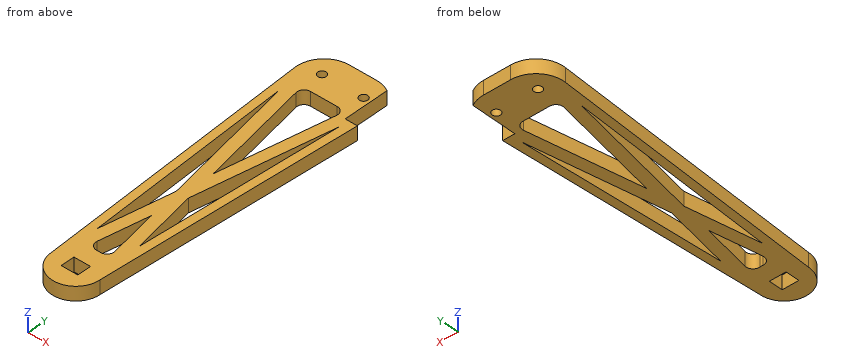
```python
from build123d import *

# Parameters (mm, degrees)
SKETCH1_R           = 3
BOSS_EXTRUDE2_DEPTH = 10
FILLET1_R           = 20
FILLET2_R           = 20
CUT_EXTRUDE1_START  = -10
CUT_EXTRUDE1_DEPTH  = 10
FILLET3_R           = 5
CUT_EXTRUDE6_DEPTH  = 10


with BuildPart() as part:
    # Sketch1 → Boss-Extrude2 (new body)
    with BuildSketch(Plane.XY):
        with BuildLine():
            Line((-30, 15.770412854), (-30, 0))
            Line((-30, 0), (-17.5, -210))
            ThreePointArc((-17.5, -210), (0, -227.5), (17.5, -210))
            Line((17.5, -210), (30, 0))
            Line((30, 0), (30, 15.770412854))
            Line((30, 15.770412854), (-30, 15.770412854))
        make_face()
        with Locations((-15, 0)):
            Circle(SKETCH1_R, mode=Mode.SUBTRACT)
        with Locations((15, 0)):
            Circle(SKETCH1_R, mode=Mode.SUBTRACT)
        Polygon((0, -205), (6, -205), (6, -215), (-6, -215), (-6, -205), align=None, mode=Mode.SUBTRACT)
    extrude(amount=BOSS_EXTRUDE2_DEPTH)

    # Fillet1
    fillet1_edges = [part.edges().sort_by_distance(p)[0] for p in [
        (-30, 15.770412854, 5),
    ]]
    fillet(fillet1_edges, radius=FILLET1_R)

    # Fillet2
    fillet2_edges = [part.edges().sort_by_distance(p)[0] for p in [
        (30, 15.770412854, 5),
    ]]
    fillet(fillet2_edges, radius=FILLET2_R)

    # Sketch4 → Cut-Extrude1 (cut)
    with BuildSketch(Plane.XY.offset(10).offset(CUT_EXTRUDE1_START)):
        Polygon((-15.651797422, -15), (0.190220551, -102.160979768), (15.643622882, -15), (15, -15), align=None)
        Polygon((-22.473027071, -25.6531452), (-13.367328465, -178.628881795), (-4.134156204, -126.551525408), align=None)
        Polygon((22.230419841, -27.161313899), (4.615986353, -126.511039477), (13.430162671, -175.005634359), align=None)
        with BuildLine():
            Line((0.291609598, -150.901585116), (-7.372445375, -194.128735111))
            ThreePointArc((-7.372445375, -194.128735111), (0.476576628, -192.506490497), (8.225632191, -194.553674383))
            Line((8.225632191, -194.553674383), (0.291609598, -150.901585116))
        make_face()
    extrude(amount=CUT_EXTRUDE1_DEPTH, mode=Mode.SUBTRACT)

    # Fillet3
    fillet3_edges = [part.edges().sort_by_distance(p)[0] for p in [
        (8.225632191, -194.553674383, 5),
        (-7.372445375, -194.128735111, 5),
        (-15.651797422, -15, 5),
        (15.643622882, -15, 5),
    ]]
    fillet(fillet3_edges, radius=FILLET3_R)

    # Sketch5 → Cut-Extrude6 (cut)
    with BuildSketch(Plane.XY.offset(10)):
        with BuildLine():
            Line((29.260488635, 0), (20, 0))
            Line((20, 0), (20, -20))
            Line((20, -20), (28.80952381, -20))
            Line((28.80952381, -20), (29.677502384, -5.417959945))
            ThreePointArc((29.677502384, -5.417959945), (29.653859351, -2.694751229), (29.260488635, 0))
        make_face()
        with BuildLine():
            Line((20, 12.921923742), (20, 0))
            Line((20, 0), (29.260488635, 0))
            ThreePointArc((29.260488635, 0), (25.96931496, 7.420606017), (20, 12.921923742))
        make_face()
    extrude(amount=-CUT_EXTRUDE6_DEPTH, mode=Mode.SUBTRACT)


solid = part.part
```
Design review of the part built by this model. Coordinates are the model's own, in mm. Give positions to 0.01 mm unless a question says otherwise; leave off trailing zeros. Loops run counter-clockwise (first coordinate to the right, second up) from the corner with the lowest first, then second, coordinate; pieces in that order, holes last. Notation, with made-up numbers: (-21.5, 10.25) -> (-7.5, 10.25) arc R7 cw to (-7.5, 14.25) -> close; hole circle Ø5 at (-18, -2.75). An arc over 180 degrees is marked (long way). One line per item, written item: value.
Q1. We need section A-A on y = -122.5. Give the boundary of the cut face in (x, z).
Numbers:
outline: (-22.71, 0) -> (-16.71, 0) -> (-16.71, 10) -> (-22.71, 10) -> close; (-4.87, 0) -> (5.33, 0) -> (5.33, 10) -> (-4.87, 10) -> close; (16.56, 0) -> (22.71, 0) -> (22.71, 10) -> (16.56, 10) -> close
Q2. For L1, parallel to X at y = -68, z = 5.25; L2, parallel to X at y = -147.5, z = 3.5; L3, parallel to X at y = -99.5, z = 9, list the stretches that pass through material, from the lowest coordinate up.
Numbers:
L1: x = -25.95 to -19.95, -14.78 to -6.02, 6.25 to 14.99, 19.8 to 25.95
L2: x = -21.22 to -15.22, -7.85 to 8.43, 15.07 to 21.22
L3: x = -24.08 to -18.08, -9.05 to -0.29, 0.66 to 9.4, 17.92 to 24.08
Q3. We need section B-B on y = -156.5. Give the boundary of the cut face in (x, z), and give its area (3 significant figures).
Numbers:
outline: (-20.68, 0) -> (-14.68, 0) -> (-14.68, 10) -> (-20.68, 10) -> close; (-9.44, 0) -> (-0.7, 0) -> (-0.7, 10) -> (-9.44, 10) -> close; (1.31, 0) -> (10.07, 0) -> (10.07, 10) -> (1.31, 10) -> close; (14.53, 0) -> (20.68, 0) -> (20.68, 10) -> (14.53, 10) -> close
area: 297 mm^2
Q4. For pin 1 Ø3 at (y, z) = (-149, 4.5) entering from -X; pin 2 Ø7 at (x, y) = (-15, 0) entering from -Z; pin 3 Ø5 at (y, z) = (-210, 7) entering from +X; pin 4 Ø3 at (x, z) = (-2, 3.5) entering from -Y, all flat-tipped, find the tip position at first contact; note any pin that passes through.
Numbers:
pin 1: stops at x = -21.22
pin 2: stops at z = 0
pin 3: stops at x = 17.65
pin 4: stops at y = -227.49
Q5. We need section C-C on z = 2. Give the number of separate pieces and of enclosed holes in the cut face, and give its area (3 significant figures).
Numbers:
separate pieces: 1
enclosed holes: 7
area: 7,330 mm^2
Q6. We need section D-D on y = -198. Give the boundary of the cut face in (x, z).
Numbers:
outline: (-18.21, 0) -> (18.21, 0) -> (18.21, 10) -> (-18.21, 10) -> close
